```python
from build123d import *

# Parameters (mm, degrees)
SKETCH_1_W          = 155
SKETCH_1_H          = 55
EXTRUDE_1_DEPTH     = 20
FILLET_1_R          = 3.5
SHELL_1_T           = -2.2
SKETCH_2_R          = 1.1
CUT_EXTRUDE_1_DEPTH = 10
EXTRUDE_START       = 3
SKETCH_3_R          = 2.75
SKETCH_3_R_2        = 1.1
EXTRUDE_2_DEPTH     = 3
SKETCH_4_R          = 0.75
SKETCH_4_W          = 10.5
SKETCH_4_H          = 9.5
SKETCH_4_W_2        = 12.5
SKETCH_4_H_2        = 11
SKETCH_4_W_3        = 15
SKETCH_4_H_3        = 2.5
CUT_EXTRUDE_2_DEPTH = 3
SKETCH_5_W          = 125
SKETCH_5_H          = 5
CUT_EXTRUDE_3_DEPTH = 3


with BuildPart() as part:
    # 草图1 → 凸台-拉伸1 (new body)
    with BuildSketch(Plane.XY):
        with Locations((77.5, -27.5)):
            Rectangle(SKETCH_1_W, SKETCH_1_H)
    extrude(amount=EXTRUDE_1_DEPTH)

    # 圆角1
    fillet_1_edges = [part.edges().sort_by_distance(p)[0] for p in [
        (0, 0, 10),
        (155, 0, 10),
        (155, -55, 10),
        (0, -55, 10),
    ]]
    fillet(fillet_1_edges, radius=FILLET_1_R)

    # 抽壳1
    shell_1_openings = [part.faces().sort_by_distance(p)[0] for p in [
        (77.5, -27.5, 20),
    ]]
    offset(amount=SHELL_1_T, openings=shell_1_openings, kind=Kind.INTERSECTION)

    # 草图2 → 切除-拉伸1 (cut)
    with BuildSketch(Plane.XY.offset(2.2)):
        with Locations((27.5, -12.5)):
            Circle(SKETCH_2_R)
        with Locations((127.5, -12.5)):
            Circle(SKETCH_2_R)
        with Locations((127.5, -42.5)):
            Circle(SKETCH_2_R)
        with Locations((27.5, -42.5)):
            Circle(SKETCH_2_R)
    extrude(amount=-CUT_EXTRUDE_1_DEPTH, mode=Mode.SUBTRACT)

    # 草图3 → 凸台-拉伸2 (add)
    # profile 1 of 8: a face of its own
    with BuildSketch(Plane.XY.offset(2.2).offset(EXTRUDE_START)):
        with Locations((27.5, -12.5)):
            Circle(SKETCH_3_R)
        with Locations((27.5, -12.5)):
            Circle(SKETCH_3_R_2, mode=Mode.SUBTRACT)
    # profile 2 of 8: a face of its own
    with BuildSketch(Plane.XY.offset(2.2).offset(EXTRUDE_START)):
        with Locations((127.5, -12.5)):
            Circle(SKETCH_3_R)
        with Locations((127.5, -12.5)):
            Circle(SKETCH_3_R_2, mode=Mode.SUBTRACT)
    # profile 3 of 8: a face of its own
    with BuildSketch(Plane.XY.offset(2.2).offset(EXTRUDE_START)):
        with Locations((127.5, -42.5)):
            Circle(SKETCH_3_R)
        with Locations((127.5, -42.5)):
            Circle(SKETCH_3_R_2, mode=Mode.SUBTRACT)
    # profile 4 of 8: a face of its own
    with BuildSketch(Plane.XY.offset(2.2).offset(EXTRUDE_START)):
        with Locations((27.5, -42.5)):
            Circle(SKETCH_3_R)
        with Locations((27.5, -42.5)):
            Circle(SKETCH_3_R_2, mode=Mode.SUBTRACT)
    # profile 5 of 8: a face of its own
    with BuildSketch(Plane.XY.offset(2.2).offset(EXTRUDE_START)):
        with Locations((6.5, -6.5)):
            Circle(SKETCH_3_R)
        with Locations((6.5, -6.5)):
            Circle(SKETCH_3_R_2, mode=Mode.SUBTRACT)
    # profile 6 of 8: a face of its own
    with BuildSketch(Plane.XY.offset(2.2).offset(EXTRUDE_START)):
        with Locations((148.5, -6.5)):
            Circle(SKETCH_3_R)
        with Locations((148.5, -6.5)):
            Circle(SKETCH_3_R_2, mode=Mode.SUBTRACT)
    # profile 7 of 8: a face of its own
    with BuildSketch(Plane.XY.offset(2.2).offset(EXTRUDE_START)):
        with Locations((148.5, -48.5)):
            Circle(SKETCH_3_R)
        with Locations((148.5, -48.5)):
            Circle(SKETCH_3_R_2, mode=Mode.SUBTRACT)
    # profile 8 of 8: a face of its own
    with BuildSketch(Plane.XY.offset(2.2).offset(EXTRUDE_START)):
        with Locations((6.5, -48.5)):
            Circle(SKETCH_3_R)
        with Locations((6.5, -48.5)):
            Circle(SKETCH_3_R_2, mode=Mode.SUBTRACT)
    extrude(amount=-EXTRUDE_2_DEPTH)

    # 草图4 → 切除-拉伸2 (cut)
    with BuildSketch(Plane.XZ.offset(55)):
        with Locations(Location((89.3, 7.5, 0), (0, 0, 270))):
            Circle(SKETCH_4_R)
        with Locations((22.75, 11.25)):
            Rectangle(SKETCH_4_W, SKETCH_4_H)
        with Locations((38.25, 12)):
            Rectangle(SKETCH_4_W_2, SKETCH_4_H_2)
        with Locations((60.3, 7.75)):
            Rectangle(SKETCH_4_W_3, SKETCH_4_H_3)
    extrude(amount=-CUT_EXTRUDE_2_DEPTH, mode=Mode.SUBTRACT)

    # 草图5 → 切除-拉伸3 (cut)
    with BuildSketch(Plane(origin=(0, 0, 0), x_dir=(1, 0, 0), z_dir=(0, 1, 0))):
        with Locations((77.5, -17.5)):
            Rectangle(SKETCH_5_W, SKETCH_5_H)
    extrude(amount=-CUT_EXTRUDE_3_DEPTH, mode=Mode.SUBTRACT)


solid = part.part
```
Work out the finished part from the listing and answer in its coordinate system (mm). A direction names the side the tool comes from. Coordinates: 2 decimals unless noted, no trailing zeros. Order: outer loops, then holes, each group sorted by start corner. A loop starts at its lowest first (then second) coordinate and runs counter-clockwise, first axis right, second up. Notation, with made-up numbers: M 84,86.25 L 90,86.25 A22 ccw 90,104.25 Z; hole C 36.25,70.25 d9. An arc over 180 degrees is marked long. Use CSV: the item, a comma, the result in double quotes.
1) Flat-ended cylindrical pins translate along their axes: pin 1 Ø2.5 at (y, z) = (-54, 12) entering from -X; pin 2 Ø1.1 at (y, z) = (-1, 18.5) entering from -X; pin 3 Ø4 at (x, y) = (103, -18.5) entering from +Z. Find the tip coordinate at first contact, or state that the pin passes through.
Worked out:
pin 1,"stops at x = 0.23"
pin 2,"stops at x = 0.59"
pin 3,"stops at z = 2.2"
2) Section B-B on y = -17 is taken. Write down the section's boundary in (x, z), plus the area to 3 significant figures.
Worked out:
outline,"M 0,0 L 155,0 L 155,20 L 152.8,20 L 152.8,2.2 L 2.2,2.2 L 2.2,20 L 0,20 Z"
area,"419 mm^2"
3) Section C-C on x = 91.5 is taken. Write down the section's boundary in (y, z), plus the area to 3 significant figures.
Worked out:
outline,"M -55,0 L 0,0 L 0,15 L -2.2,15 L -2.2,2.2 L -52.8,2.2 L -52.8,20 L -55,20 Z"
area,"188 mm^2"
4) For faces 1 (the face through (2.2, -28, 11)), 2 (the face through (76, -55, 10)), determine the directions among +Z, -Z, +X, -X, +Y, -Y from which every point of the face is accessible in a straight line to the end or side of a thin tool.
Worked out:
face 1,"+Z"
face 2,"+Z, -Z, +X, -X, -Y"
5) Determine the mould class of faces 3 (the face through (76, -52.8, 11)), 4 (the face through (76, 0, 8)), 5 (the face through (6, -50, 5.2)), 6 (the face through (77, -54, 20)) for opening direction Y: released by +Y, released by -Y, zero draft, split by the parting line, or undercut.
Worked out:
face 3,"undercut"
face 4,"released by +Y"
face 5,"undercut"
face 6,"zero draft"
6) Section A-A on z = 12 is taken. Write down the section's boundary in (x, y).
Worked out:
outline,"M 0,-51.5 A3.5 ccw 3.5,-55 L 17.5,-55 L 17.5,-52.8 L 3.5,-52.8 A1.3 cw 2.2,-51.5 L 2.2,-3.5 A1.3 cw 3.5,-2.2 L 151.5,-2.2 A1.3 cw 152.8,-3.5 L 152.8,-51.5 A1.3 cw 151.5,-52.8 L 44.5,-52.8 L 44.5,-55 L 151.5,-55 A3.5 ccw 155,-51.5 L 155,-3.5 A3.5 ccw 151.5,0 L 3.5,0 A3.5 ccw 0,-3.5 Z; M 28,-55 L 32,-55 L 32,-52.8 L 28,-52.8 Z"
7) Consider line 1 (Y direction, x = 27.5, z = 2.85); line 2 (Y direction, x = 6.5, z = 2.95); line 3 (Y direction, x = 78, z = 3.75). Determine where each line is inside the solid, lowest interval first. Write a range as [from, to].
Worked out:
line 1,"y = [-55, -52.8], [-45.25, -43.6], [-41.4, -39.75], [-15.25, -13.6], [-11.4, -9.75], [-2.2, 0]"
line 2,"y = [-55, -52.8], [-51.25, -49.6], [-47.4, -45.75], [-9.25, -7.6], [-5.4, -3.75], [-2.2, 0]"
line 3,"y = [-55, -52.8], [-2.2, 0]"
